Source: CAD feature listing. Evaluate the final solid. Frame: model axes, mm. A direction names the side the tool comes from. Give positions to 0.01 mm unless a question says otherwise; leave off trailing zeros. Write each loop counter-clockwise with the first axis right and the second up, starting at its lowest first coordinate (ties: lowest second). Pieces come first, ordered by that corner, then holes. Notation, with made-up numbers: (-7.75, 34.25) -> (41.25, 34.25) arc R24 cw to (41.25, 65.25) -> close; hole circle Ø7 at (-21.75, 36). An arc over 180 degrees is marked (long way). Write item = value, one per line.
from build123d import *

# Parameters (mm, degrees)
F0_R     = 5
F1_DEPTH = 5


with BuildPart() as f1:
    # F0 (on Front) → F1 (new body)
    with BuildSketch(Plane.XZ):
        with BuildLine():
            Line((54.568551, 10), (-38.631449, 10))
            ThreePointArc((-38.631449, 10), (-47.631449, 1), (-38.631449, -8))
            Line((-38.631449, -8), (54.568551, -8))
            Line((54.568551, -8), (54.568551, 10))
        make_face()
        with Locations((-38.631449, 0)):
            Circle(F0_R, mode=Mode.SUBTRACT)
        with BuildLine():
            ThreePointArc((29.568551, 2.75), (32.318551, 0), (29.568551, -2.75))
            Line((29.568551, -2.75), (-22.631449, -2.75))
            ThreePointArc((-22.631449, -2.75), (-25.381449, 0), (-22.631449, 2.75))
            Line((-22.631449, 2.75), (29.568551, 2.75))
        make_face(mode=Mode.SUBTRACT)
    extrude(amount=F1_DEPTH)


solid = f1.part
1) Draft query along Z for faces 1 (the flat face through (3, -2, 2.75)), 2 (the flat face through (3, -5, 3)), 3 (the flat face through (7, -2, -8)). Return one class per face: pulls with the +Z half, pulls with the -Z half, needs draft (parallel to the pull), parting line crosses it, or undercut.
Computed:
face_1 = undercut
face_2 = needs draft
face_3 = pulls with the -Z half
2) Contact query for flat-ended pins moving along their axis: pin 1 (1 mm diameter, centred on y = -0.5, z = -3, fed in from -X); pin 2 (1 mm diameter, centred on x = 28, z = 3.5, fed in from +Y). Output: stop coordinate, or through.
Computed:
pin_1 = -46.92
pin_2 = 0
3) Access query for faces 4 (the cylindrical face through (-25.38, -2.46, -0.06)), 5 (the cylindrical face through (-47.63, -2.46, 1.2)). Directions: +Z, -Z, +X, -X, +Y, -Y. A direction counts if a zero-diameter tool reaches every point of the face in a straight line with its end or side. Return the directions, or none.
Computed:
face_4 = +Y, -Y
face_5 = -X, +Y, -Y
4) Cut plane B-B (x = -12.5). Return the cut outline in (y, z), then the cut area to 3 significant figures.
Computed:
outline = (-5, -8) -> (0, -8) -> (0, -2.75) -> (-5, -2.75) -> close; (-5, 2.75) -> (0, 2.75) -> (0, 10) -> (-5, 10) -> close
area = 62.5 mm²
5) Cut plane C-C (z = 1). Return the cut outline in (x, y).
Computed:
outline = (-47.63, -5) -> (-43.53, -5) -> (-43.53, 0) -> (-47.63, 0) -> close; (-33.73, -5) -> (-25.19, -5) -> (-25.19, 0) -> (-33.73, 0) -> close; (32.13, -5) -> (54.57, -5) -> (54.57, 0) -> (32.13, 0) -> close
6) Cut plane D-D (x = -40). Return the cut outline in (y, z).
Computed:
outline = (-5, -7.9) -> (0, -7.9) -> (0, -4.81) -> (-5, -4.81) -> close; (-5, 4.81) -> (0, 4.81) -> (0, 9.9) -> (-5, 9.9) -> close
7) Cut plane A-A (y = -2.9). Return the cut outline in (x, z), then the cut area to 3 significant figures.
Computed:
outline = (-38.63, -8) -> (54.57, -8) -> (54.57, 10) -> (-38.63, 10) arc R9 ccw to start; hole circle Ø10 at (-38.63, 0); hole (-22.63, -2.75) -> (29.57, -2.75) arc R2.75 ccw to (29.57, 2.75) -> (-22.63, 2.75) arc R2.75 ccw to start
area = 1,420 mm²
8) Material intervals for L1, parallel to Z at x = 2, y = -1.55; L2, parallel to X at y = -2.5, z = 2.5; L3, parallel to X at y = -3.1, z = 2.25, sorted ascending.
Computed:
L1 = -8 to -2.75, 2.75 to 10
L2 = -47.51 to -42.96, -34.3 to -23.78, 30.71 to 54.57
L3 = -47.54 to -43.1, -34.17 to -24.21, 31.15 to 54.57
